```python
from build123d import *

# Parameters (mm, degrees)
PAD079_DEPTH    = 25
SKETCH168_R     = 28
POCKET096_DEPTH = 25
SKETCH169_W     = 48.856676
SKETCH169_H     = 39
PAD080_DEPTH    = 25
SKETCH172_W     = 27
SKETCH172_H     = 39
PAD081_DEPTH    = 12
SKETCH175_W     = 27
SKETCH175_H     = 6
PAD082_DEPTH    = 15
SKETCH170_W     = 40.975294
SKETCH170_H     = 39
POCKET097_DEPTH = 25.001
PAD083_DEPTH    = 27
POCKET098_DEPTH = 9
SKETCH177_R     = 6
POCKET099_DEPTH = 14
SKETCH171_R     = 2.65
POCKET100_DEPTH = 55.429338
SKETCH174_R     = 3.5
POCKET101_DEPTH = 8
SKETCH176_R     = 1.5
POCKET102_DEPTH = 6


with BuildPart() as part:
    # Sketch167 → Pad079 (new body)
    with BuildSketch(Plane.XY):
        with BuildLine():
            ThreePointArc((24.428333, -19.085506), (0, 31), (-24.428333, -19.085506))
            Line((-24.428333, -19.085506), (24.428333, -19.085506))
        make_face()
    extrude(amount=PAD079_DEPTH)

    # Sketch168 → Pocket096 (cut)
    with BuildSketch(Plane.XY):
        Circle(SKETCH168_R)
    extrude(amount=POCKET096_DEPTH, mode=Mode.SUBTRACT)

    # Sketch169 → Pad080 (join)
    with BuildSketch(Plane.XY):
        with Locations((0, -38.5855)):
            Rectangle(SKETCH169_W, SKETCH169_H)
    extrude(amount=PAD080_DEPTH)

    # Sketch172 (on Face3 of Pad080) → Pad081 (join)
    with BuildSketch(Plane(origin=(-24.428338, 0, 0), x_dir=(0, -1, 0), z_dir=(-1, 0, 0))):
        with Locations((32.5855, 5.5)):
            Rectangle(SKETCH172_W, SKETCH172_H)
    extrude(amount=PAD081_DEPTH)

    # Sketch175 → Pad082 (join)
    with BuildSketch(Plane(origin=(-34.852298, 0, 0), x_dir=(0, -1, 0), z_dir=(-1, 0, 0))):
        with Locations((32.5855, -11)):
            Rectangle(SKETCH175_W, SKETCH175_H)
    extrude(amount=PAD082_DEPTH)

    # Sketch170 → Pocket097 (cut, through all)
    with BuildSketch(Plane.XY):
        with Locations((0, -38.5855)):
            Rectangle(SKETCH170_W, SKETCH170_H)
    extrude(amount=POCKET097_DEPTH, mode=Mode.SUBTRACT)

    # Sketch178 (on Face3 of Pocket097) → Pad083 (join)
    with BuildSketch(Plane(origin=(-2e-06, -19.085505, 0), x_dir=(-1, 0, 0), z_dir=(0, 1, 0))):
        with BuildLine():
            ThreePointArc((36.284298, -3.912067), (37.350001, -6.635466), (39.740093, -8.32072))
            Line((34.729457, -10.005197), (39.740093, -8.32072))
            Line((36.284298, -3.912067), (34.729457, -10.005197))
        make_face()
    extrude(amount=-PAD083_DEPTH)

    # Sketch173 → Pocket098 (cut)
    with BuildSketch(Plane(origin=(-20.254085, -4e-06, 0), x_dir=(0, 1, 0), z_dir=(1, 0, 0))):
        with BuildLine():
            Line((-43.0855, 21.332453), (-43.0855, 4.527547))
            ThreePointArc((-43.0855, 4.527547), (-42.110884, 2.174616), (-39.757953, 1.2))
            Line((-39.757953, 1.2), (-22.878191, 1.2))
            ThreePointArc((-22.878191, 1.2), (-20.90346, 2.01796), (-20.0855, 3.992691))
            Line((-20.0855, 3.992691), (-20.0855, 21.342255))
            ThreePointArc((-20.0855, 21.342255), (-20.922514, 23.362986), (-22.943245, 24.2))
            Line((-22.943245, 24.2), (-40.217953, 24.2))
            ThreePointArc((-40.217953, 24.2), (-42.245615, 23.360115), (-43.0855, 21.332453))
        make_face()
    extrude(amount=-POCKET098_DEPTH, mode=Mode.SUBTRACT)

    # Sketch177 → Pocket099 (cut)
    with BuildSketch(Plane(origin=(0, 0, -14), x_dir=(1, 0, 0), z_dir=(0, 0, -1))):
        with Locations((-24.428338, 46.0855)):
            Circle(SKETCH177_R)
        with Locations((-24.428338, 19.0855)):
            Circle(SKETCH177_R)
    extrude(amount=-POCKET099_DEPTH, mode=Mode.SUBTRACT)

    # Sketch171 (on Face12 of Pocket099) → Pocket100 (cut, through all)
    with BuildSketch(Plane(origin=(-24.428338, 0, 0), x_dir=(0, -1, 0), z_dir=(-1, 0, 0))):
        with Locations((52.5, 19)):
            Circle(SKETCH171_R)
        with Locations((52.5, 6)):
            Circle(SKETCH171_R)
    extrude(amount=-POCKET100_DEPTH, mode=Mode.SUBTRACT)

    # Sketch174 (on Face7 of Pocket100) → Pocket101 (cut)
    with BuildSketch(Plane(origin=(-36.428338, 0, 0), x_dir=(0, -1, 0), z_dir=(-1, 0, 0))):
        with Locations((32, 12.5)):
            Circle(SKETCH174_R)
    extrude(amount=-POCKET101_DEPTH, mode=Mode.SUBTRACT)

    # Sketch176 (on Face10 of Pocket101) → Pocket102 (cut)
    with BuildSketch(Plane(origin=(0, 0, -14), x_dir=(1, 0, 0), z_dir=(0, 0, -1))):
        with Locations((-44, 38.8542)):
            Circle(SKETCH176_R)
        with Locations((-44, 25.8542)):
            Circle(SKETCH176_R)
        with Locations((-41, 32.3542)):
            Circle(SKETCH176_R)
    extrude(amount=-POCKET102_DEPTH, mode=Mode.SUBTRACT)


solid = part.part
```
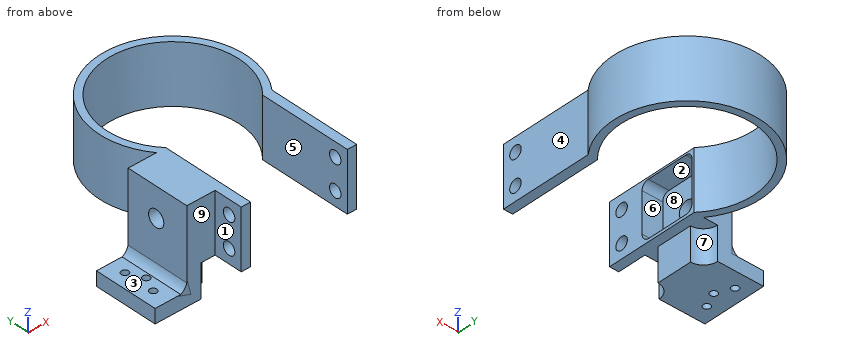
Geometry check sheet. Reference: the model listing, model coordinates, mm. Face numbers are marked on the shaded views. A direction names the side the tool comes from. Give positions to 0.01 mm unless a question says otherwise; leave off trailing zeros. Write each loop counter-clockwise with the first axis right and the second up, starting at its lowest first coordinate (ties: lowest second). Pieces come first, ordered by that corner, then holes.
1) Release check for a two-part mould opening along X. For the marked faces 6, 7, 8 and 9 record: pulls with the +X half, pulls with the -X half, needs draft (parallel to the pull), parting line crosses it, or undercut.
2) Section check B-B, the plane z = 19. Record the boundary of the cut face in (x, y), and give its area (3 significant figures).
3) Access from +Z, -Z, +X, -X, +Y, -Y to the whole of each face (thin tool, end or side, straight path). Record for the marked faces 1, 2, 3, 4 and 5.
4) Material ranges on L1, parallel to Y at x = -44, z = -11; L2, parallel to X at y = 0, z = 6; L3, parallel to Z at x = -21, y = -31, recorded low to high.
5) Gauge pin test, flat ends, axial feed: pin 1 (2.5 mm diameter, centred on x = -36, z = -5.5, fed in from -Y); pin 2 (4 mm diameter, centred on x = -44, y = -25.85, fed in from +Z); pin 3 (1.3 mm diameter, centred on x = -38, z = -7, fed in from +Y). Record the tip position at first contact, or that the pin passes through.
6) Section check D-D, the plane y = 2.5. Record the boundary of the cut face in (x, z), and give its area (3 significant figures).
7) Section check A-A, the plane y = -52.5. Record the boundary of the cut face in (x, z), and give its area (3 significant figures).
8) Section check C-C, the plane x = -41. Record the boundary of the cut face in (y, z).
Computed:
1. face 6: undercut
1. face 7: pulls with the +X half
1. face 8: undercut
1. face 9: needs draft
2. outline: (-36.43, -46.09) - (-24.43, -46.09) - (-24.43, -49.85) - (-20.49, -49.85) - (-20.49, -43.09) - (-29.25, -43.09) - (-29.25, -20.09) - (-20.49, -20.09) - (-20.49, -19.09) arc R28 cw (long way) to (20.49, -19.09) - (20.49, -49.85) - (24.43, -49.85) - (24.43, -19.09) arc R31 ccw (long way) to (-24.43, -19.09) - (-36.43, -19.09) - close; (-24.43, -58.09) - (-20.49, -58.09) - (-20.49, -55.15) - (-24.43, -55.15) - close; (20.49, -58.09) - (24.43, -58.09) - (24.43, -55.15) - (20.49, -55.15) - close
2. area: 791 mm2
3. face 1: +Z, -Z, -X, -Y
3. face 2: none
3. face 3: +Z, -X, +Y, -Y
3. face 4: +Z, -Z, +X, -Y
3. face 5: +Z, -Z, -Y
4. L1: y = -46.09 to -40.35, -37.35 to -27.35, -24.35 to -19.09
4. L2: x = -31 to -28, 28 to 31
4. L3: z = 0 to 1.2, 24.2 to 25
5. pin 1: stops at y = -46.09
5. pin 2: stops at z = -8
5. pin 3: stops at y = -19.09
6. outline: (-30.9, 0) - (-27.89, 0) - (-27.89, 25) - (-30.9, 25) - close; (27.89, 0) - (30.9, 0) - (30.9, 25) - (27.89, 25) - close
6. area: 151 mm2
7. outline: (-24.43, 0) - (-20.49, 0) - (-20.49, 3.35) - (-24.43, 3.35) - close; (-24.43, 8.65) - (-20.49, 8.65) - (-20.49, 16.35) - (-24.43, 16.35) - close; (-24.43, 21.65) - (-20.49, 21.65) - (-20.49, 25) - (-24.43, 25) - close; (20.49, 0) - (24.43, 0) - (24.43, 3.35) - (20.49, 3.35) - close; (20.49, 8.65) - (24.43, 8.65) - (24.43, 16.35) - (20.49, 16.35) - close; (20.49, 21.65) - (24.43, 21.65) - (24.43, 25) - (20.49, 25) - close
7. area: 113 mm2
8. outline: (-46.09, -14) - (-33.85, -14) - (-33.85, -8) - (-46.09, -8) - close; (-30.85, -14) - (-19.09, -14) - (-19.09, -8) - (-30.85, -8) - close
